Input: dimensioned drawing with shaded views. Units: mm. Origin: part minimum x, y, z. A direction names the side the tool comes from. Round coordinates to 2 decimals unless told otherwise and drop trailing zeros. Loops run counter-clockwise (first coordinate to the right, second up) from the corner with the lowest first, then second, coordinate; pieces in that order, holes last. Notation, with made-up numbers: (24.25, 19.5) - (34.25, 19.5) arc R21 cw to (34.25, 31.5) - close; hole circle Ø5 at (48, 87.25). An arc over 180 degrees is marked (long way). Use CSV: the item, a comma, the result in double quotes. Start each with the question number.
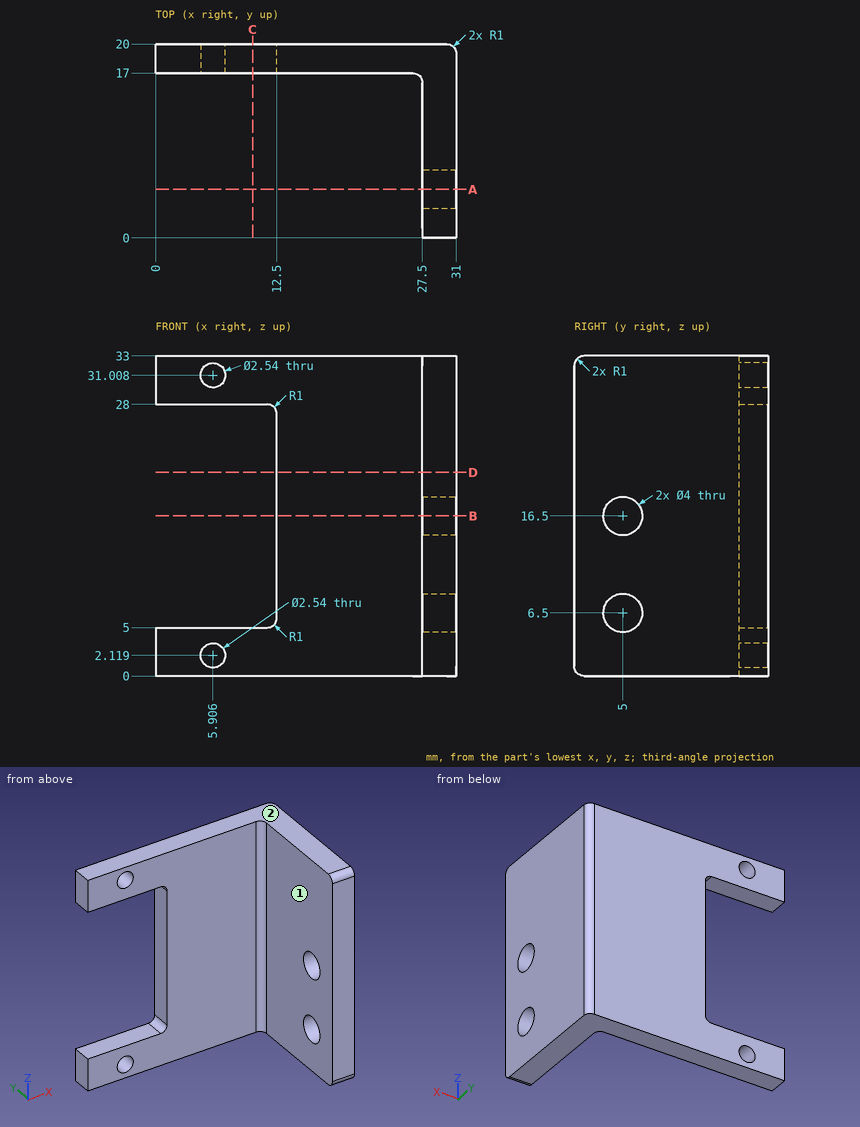
1. Reachability of the marked faces 1 and 2 from +Z, -Z, +X, -X, +Y, -Y: full face, straight path, thin tool, end or side. Return the list, or none.
2. Section query A-A on y = 5. Return the cut outline in (x, z).
3. Section query D-D on z = 21. Return the cut outline in (x, y).
4. Contact query for flat-ended pins moving along their axis: P1, Ø0.9, axis at y = 19, z = 17, coming from the -X side; P2, Ø5, axis at y = 9.5, z = 23, coming from the -X side; P3, Ø3.5, axis at x = 5.91, z = 31.01, coming from the -Y side. Output: stop coordinate, or through.
5. Line query: line 1 along Y through (x, z) = (14, 6); line 2 along X through (y, z) = (9.5, 5.5); line 3 along Y through (x, z) = (29.9, 6.5). Output: solid intervals per line, ascending.
6. Section query B-B on z = 16.5. Return the cut outline in (x, y).
7. Section query C-C on x = 10. Return the cut outline in (y, z), and give its area (3 significant figures).
Values:
1,face 1,"+Z, -Z, -X, -Y"
1,face 2,"+Z, +X, -X, +Y, -Y"
2,outline,"(27.5, 0) - (31, 0) - (31, 4.5) - (27.5, 4.5) - close; (27.5, 8.5) - (31, 8.5) - (31, 14.5) - (27.5, 14.5) - close; (27.5, 18.5) - (31, 18.5) - (31, 33) - (27.5, 33) - close"
3,outline,"(12.5, 17) - (26.5, 17) arc R1 cw to (27.5, 16) - (27.5, 0) - (31, 0) - (31, 19) arc R1 ccw to (30, 20) - (12.5, 20) - close"
4,P1,"stops at x = 12.5"
4,P2,"stops at x = 27.5"
4,P3,"stops at y = 17"
5,line 1,"y = 17 to 20"
5,line 2,"x = 27.5 to 31"
5,line 3,"y = 0 to 3, 7 to 20"
6,outline,"(12.5, 17) - (26.5, 17) arc R1 cw to (27.5, 16) - (27.5, 7) - (31, 7) - (31, 19) arc R1 ccw to (30, 20) - (12.5, 20) - close; (27.5, 0) - (31, 0) - (31, 3) - (27.5, 3) - close"
7,outline,"(17, 0) - (20, 0) - (20, 5) - (17, 5) - close; (17, 28) - (20, 28) - (20, 33) - (17, 33) - close"
7,area,"30.0 mm^2"
